Geometry check sheet. Reference: the model listing, model coordinates, mm. A direction names the side the tool comes from. Give positions to 0.01 mm unless a question says otherwise; leave off trailing zeros. Order: outer loops, then holes, each group sorted by start corner. A loop starts at its lowest first (then second) coordinate and runs counter-clockwise, first axis right, second up. Notation, with made-up numbers: M -37.75,-17.5 L -14.75,-17.5 A22 cw -14.75,16.5 Z; hole C 20,-15 d10. An arc over 180 degrees is marked long. Answer as CSV lines item,"result". Start each with the question number.
```python
from build123d import *

# Parameters (mm, degrees)
SKETCH_1_W               = 30
SKETCH_1_H               = 30
EXTRUDE_1_DEPTH          = 30
CUT_EXTRUDE_8_DEPTH      = 52.961524227
CUT_EXTRUDE_9_DEPTH      = 47.904157598
CUT_EXTRUDE_9_DEPTH_BACK = 47.904157598
SKETCH_16_W              = 20
SKETCH_16_H              = 10
CUT_EXTRUDE_10_DEPTH     = 52.961524227


with BuildPart() as part:
    # 草圖1 → 填料-伸1 (new body)
    with BuildSketch(Plane.XY):
        with Locations((15, 15)):
            Rectangle(SKETCH_1_W, SKETCH_1_H)
    extrude(amount=-EXTRUDE_1_DEPTH)

    # 草圖11 → 除料-伸長8 (cut, through all)
    with BuildSketch(Plane.XY):
        Polygon((10, 30), (10, 20), (20, 20), (20, 10), (30, 10), (30, 30), align=None)
    extrude(amount=-CUT_EXTRUDE_8_DEPTH, mode=Mode.SUBTRACT)

    # 草圖16 → 除料-伸長9 (cut, two sides: drawn at the far end of the back side and taken through both)
    with BuildSketch(Plane(origin=(0, 10, 0), x_dir=(1, 0, 0), z_dir=(0, 1, 0)).offset(-CUT_EXTRUDE_9_DEPTH_BACK)):
        with Locations((20, 5)):
            Rectangle(SKETCH_16_W, SKETCH_16_H)
    extrude(amount=CUT_EXTRUDE_9_DEPTH + CUT_EXTRUDE_9_DEPTH_BACK, mode=Mode.SUBTRACT)

    # 草圖20 → 除料-伸長10 (cut, through all)
    with BuildSketch(Plane(origin=(30, 0, 0), x_dir=(0, 0, -1), z_dir=(1, 0, 0))):
        Polygon((0, 30), (0, 10), (20, 30), align=None)
    extrude(amount=-CUT_EXTRUDE_10_DEPTH, mode=Mode.SUBTRACT)


solid = part.part
```
Item 1: Scan lines: line 1 along X through (y, z) = (28.5, -27.75); line 2 along Y through (x, z) = (16.5, -16). Record each from-to range of solid material in increasing order.
Item 2: Section check A-A on z = -22.5. Record the boundary of the cut face in (x, y).
Item 3: Section check D-D on z = -14. Record the boundary of the cut face in (x, y), then the cut area to 3 significant figures.
Item 4: Section check B-B on x = 7.5. Record the boundary of the cut face in (y, z).
Item 5: Section check C-C on y = 11.5. Record the boundary of the cut face in (x, z), then the cut area to 3 significant figures.
Item 6: Depth check by flat-ended pin: pin 1 Ø4 at (y, z) = (21.5, -17) entering from -X; pin 2 Ø8 at (y, z) = (9.5, -3.5) entering from +X; pin 3 Ø10 at (x, y) = (18, 6.5) entering from +Z; pin 4 Ø11 at (y, z) = (17, -18) entering from +X. Enter the tip coordinate at first touch or a pass-through.
Item 7: Access from +Z, -Z, +X, -X, +Y, -Y to the whole of each face (thin tool, end or side, straight path). Record for faces 1 (the face through (10, 8, -5)), 2 (the face through (10, 25, -22)), 3 (the face through (30, 5, -20)).
Numbers:
1,line 1,"0 to 10"
1,line 2,"0 to 20"
2,outline,"M 0,0 L 30,0 L 30,10 L 20,10 L 20,20 L 10,20 L 10,30 L 0,30 Z"
3,outline,"M 0,0 L 30,0 L 30,10 L 20,10 L 20,20 L 10,20 L 10,24 L 0,24 Z"
3,area,"540 mm2"
4,outline,"M 0,-30 L 30,-30 L 30,-20 L 10,0 L 0,0 Z"
5,outline,"M 0,-30 L 20,-30 L 20,-10 L 10,-10 L 10,-1.5 L 0,-1.5 Z"
5,area,"485 mm2"
6,pin 1,"x = 0"
6,pin 2,"x = 10"
6,pin 3,"z = -10"
6,pin 4,"x = 20"
7,face 1,"+Z, +X, +Y, -Y"
7,face 2,"+Z, -Z, +X, +Y"
7,face 3,"+Z, -Z, +X, +Y, -Y"
